Read the model definition and answer for the solid it produces. Units are mm, in the model's axes. A direction names the side the tool comes from. Give positions to 0.01 mm unless a question says otherwise; leave off trailing zeros. Order: outer loops, then holes, each group sorted by start corner. A loop starts at its lowest first (then second) coordinate and runs counter-clockwise, first axis right, second up. Notation, with made-up numbers: M 24,84 L 46,84 A29 cw 46,109 Z; hole C 62,76.5 d9. An arc over 180 degrees is marked long. Write item = value, one per line. Start each with the question number.
from build123d import *

# Parameters (mm, degrees)
BOSS_EXTRUDE1_DEPTH = 180
SKETCH3_W           = 14
SKETCH3_H           = 6.4
CUT_EXTRUDE1_DEPTH  = 7


with BuildPart() as part:
    # Sketch2 → Boss-Extrude1 (new body)
    with BuildSketch(Plane(origin=(0, 0, 0), x_dir=(1, 0, 0), z_dir=(0, 1, 0))):
        with BuildLine():
            Line((-9.16515139, 4), (9.16515139, 4))
            ThreePointArc((9.16515139, 4), (0, -10), (-9.16515139, 4))
        make_face()
    extrude(amount=BOSS_EXTRUDE1_DEPTH)

    # Sketch3 → Cut-Extrude1 (cut)
    with BuildSketch(Plane(origin=(0, 0, -4), x_dir=(-1, 0, 0), z_dir=(0, 0, -1))):
        with Locations((-0.07756818, 173.8)):
            Rectangle(SKETCH3_W, SKETCH3_H)
        with Locations((-0.07756818, 163.8)):
            Rectangle(SKETCH3_W, SKETCH3_H)
        with Locations((-0.07756818, 153.8)):
            Rectangle(SKETCH3_W, SKETCH3_H)
        with Locations((-0.07756818, 143.8)):
            Rectangle(SKETCH3_W, SKETCH3_H)
        with Locations((-0.07756818, 133.8)):
            Rectangle(SKETCH3_W, SKETCH3_H)
        with Locations((-0.07756818, 123.8)):
            Rectangle(SKETCH3_W, SKETCH3_H)
        with Locations((-0.07756818, 113.8)):
            Rectangle(SKETCH3_W, SKETCH3_H)
        with Locations((-0.07756818, 103.8)):
            Rectangle(SKETCH3_W, SKETCH3_H)
        with Locations((-0.07756818, 93.8)):
            Rectangle(SKETCH3_W, SKETCH3_H)
        with Locations((-0.07756818, 83.8)):
            Rectangle(SKETCH3_W, SKETCH3_H)
        with Locations((-0.07756818, 73.8)):
            Rectangle(SKETCH3_W, SKETCH3_H)
        with Locations((-0.07756818, 63.8)):
            Rectangle(SKETCH3_W, SKETCH3_H)
        with Locations((-0.07756818, 53.8)):
            Rectangle(SKETCH3_W, SKETCH3_H)
        with Locations((-0.07756818, 43.8)):
            Rectangle(SKETCH3_W, SKETCH3_H)
    extrude(amount=-CUT_EXTRUDE1_DEPTH, mode=Mode.SUBTRACT)


solid = part.part
1) Find section B-B on y = 134. Determine the outline of the cut face in (x, z).
2) For a pull along X with two mould halves and no side action, classify faces 3 (the face through (0, 124, 3)), 4 (the face through (0, 89, -4)) as pulls with the +X half, pulls with the -X half, needs draft (parallel to the pull), parting line crosses it, or undercut.
3) Find section C-C on z = 8. Determine the outline of the cut face in (x, y).
4) Find section D-D on y = 28.5. Determine the outline of the cut face in (x, z).
5) Find section A-A on z = 0. Count the separate pieces of the cut face and the enclosed holes in it, plus the area to 3 significant figures.
6) For faces 1 (the face through (0, 117, -1)), 2 (the face through (0, 0, 1)), determine the directions among +Z, -Z, +X, -X, +Y, -Y from which every point of the face is accessible in a straight line to the end or side of a thin tool.
7) Find the intervals of material crossed by probe 1 along X at (y, z) = (84, 0); probe 2 along X at (y, z) = (43, -2.5); probe 3 along X at (y, z) = (15, 0.5), in increasing order. Write a range as [from, to].
8) Each of these flat-tipped pins is pushed along its axis until it touches: P1, Ø10, axis at x = -6.5, y = 141.5, coming from the -Z side; P2, Ø1.9, axis at y = 84, z = -1.5, coming from the +X side; P3, Ø1, axis at y = 74, z = 6, coming from the -X side; P4, Ø1.5, axis at x = -4, y = 147.5, coming from the +Z side. Where does it stop, or does it pass through?
Numbers:
q1.outline = M -9.17,-4 L -6.92,-4 L -6.92,3 L 7.08,3 L 7.08,-4 L 9.17,-4 A10 ccw long Z
q2.face_3 = undercut
q2.face_4 = needs draft
q3.outline = M -6,0 L 6,0 L 6,180 L -6,180 Z
q4.outline = M -9.17,-4 L 9.17,-4 A10 ccw long Z
q5.separate_pieces = 1
q5.enclosed_holes = 14
q5.area = 2,350 mm2
q6.face_1 = -Z
q6.face_2 = +Z, -Z, +X, -X, -Y
q7.probe_1 = [-10, -6.92], [7.08, 10]
q7.probe_2 = [-9.68, -6.92], [7.08, 9.68]
q7.probe_3 = [-9.99, 9.99]
q8.P1 = -4
q8.P2 = 9.98
q8.P3 = -8.35
q8.P4 = 9.46
